Geometry: final body of the model. Coordinates: model frame, mm. A direction names the side the tool comes from. Coordinates: 2 decimals unless noted, no trailing zeros. Write each loop counter-clockwise with the first axis right and the second up, starting at its lowest first coordinate (ties: lowest second). Pieces come first, ordered by that corner, then holes. Notation, with made-up numbers: M 66,43.5 L 90,43.5 A18 ccw 90,57.5 Z; hole C 26.5,29.5 d8. An arc over 180 degrees is marked long. Write item = value, one per line. Start each with the question number.
Item 1: Section B-B on z = 11.5. Give the number of separate pieces and of enclosed holes in the cut face, plus the area to 3 significant figures.
Item 2: Section D-D on x = 18.5. Output: boundary loops of the cut face in (y, z).
Item 3: Pull-direction query (Y, two-part tool) for faces 1 (the flat face through (-7, 13, 15.773)), 2 (the cylindrical face through (29.887, 13.298, 7.776)), 3 (the cylindrical face through (-1.58, 19.27, 7.78)); classes: +Y half, -Y half, draft (parallel to the pull), parting line (faces both ways), or undercut.
Item 4: Reachability of faces 4 (the flat face through (-32, 17.234, 20)), 5 (the flat face through (-14.267, 36.465, 7.776)) from +Z, -Z, +X, -X, +Y, -Y: full face, straight path, thin tool, end or side. Return the list, or none.
Item 5: First-contact query: pin 1 Ø1.5 at (y, z) = (35, 12.5) entering from -X; pin 2 Ø2 at (x, y) = (15.5, 28) entering from +Z; pin 3 Ø5.5 at (x, z) = (-33, 19.5) entering from -Y; pin 4 Ø12 at (x, y) = (-44.5, 19) entering from -Z. Flat tips, straight axial feed; report the tip coordinate or a pass-through.
Item 6: Ray query, L1, parallel to X at y = 13, z = 27; L2, parallel to X at y = 14, z = 7.5; L3, parallel to Z at x = -22, y = -3. Return the intervals inside material, ascending. Write a range as [from, to].
from build123d import *

# Parameters (mm, degrees)
F1_DEPTH = 40.2336
F0_R     = 10.16
F2_DEPTH = 15.7734
F3_R     = 3.302


with BuildPart() as f1:
    # F0 (on Top) → F1 (new body)
    with BuildSketch(Plane.XY):
        with BuildLine():
            ThreePointArc((-42.827169, -15.683244), (-26.084127, -5.852856), (-19.488047, 12.407968))
            ThreePointArc((-19.488047, 12.407968), (-26.084127, 30.668792), (-42.827169, 40.49918))
            ThreePointArc((-42.827169, 40.49918), (-76.638047, 12.407968), (-42.827169, -15.683244))
        make_face()
        with BuildLine():
            ThreePointArc((-34.615282, 7.581968), (-62.350547, 12.407968), (-34.615282, 17.233968))
            Line((-34.615282, 17.233968), (-29.533747, 17.233968))
            Line((-29.533747, 17.233968), (-29.533747, 7.581968))
            Line((-29.533747, 7.581968), (-34.615282, 7.581968))
        make_face(mode=Mode.SUBTRACT)
    extrude(amount=F1_DEPTH)

    # F0 (on Top) → F2 (join)
    with BuildSketch(Plane.XY):
        with BuildLine():
            ThreePointArc((-42.827169, -15.683244), (-26.084127, -5.852856), (-19.488047, 12.407968))
            ThreePointArc((-19.488047, 12.407968), (-26.084127, 30.668792), (-42.827169, 40.49918))
            ThreePointArc((-42.827169, 40.49918), (-76.638047, 12.407968), (-42.827169, -15.683244))
        make_face()
        with BuildLine():
            ThreePointArc((-34.615282, 7.581968), (-62.350547, 12.407968), (-34.615282, 17.233968))
            Line((-34.615282, 17.233968), (-29.533747, 17.233968))
            Line((-29.533747, 17.233968), (-29.533747, 7.581968))
            Line((-29.533747, 7.581968), (-34.615282, 7.581968))
        make_face(mode=Mode.SUBTRACT)
        with BuildLine():
            ThreePointArc((-42.827169, 40.49918), (-26.084127, 30.668792), (-19.488047, 12.407968))
            ThreePointArc((-19.488047, 12.407968), (-26.084127, -5.852856), (-42.827169, -15.683244))
            Line((-42.827169, -15.683244), (13.505259, -5.183529))
            ThreePointArc((13.505259, -5.183529), (29.890809, 13.679218), (13.505259, 32.541964))
            Line((13.505259, 32.541964), (-42.827169, 40.49918))
        make_face()
        with Locations((5.911953, 12.407968)):
            Circle(F0_R, mode=Mode.SUBTRACT)
    extrude(amount=F2_DEPTH)

    # F3
    f3_edges = [f1.edges().sort_by_distance(p)[0] for p in [
        (-53.298926, 40.49918, 40.2336),
    ]]
    fillet(f3_edges, radius=F3_R)


solid = f1.part
Responses:
q1.separate_pieces = 1
q1.enclosed_holes = 2
q1.area = 3,680 mm²
q2.outline = M -3.76,0 L 31.12,0 L 31.12,15.77 L -3.76,15.77 Z
q3.face_1 = draft
q3.face_2 = parting line
q3.face_3 = undercut
q4.face_4 = +Z, -Z
q4.face_5 = +Z, -Z, +X, +Y
q5.pin_1 = -66.49
q5.pin_2 = 15.77
q5.pin_3 = -13.38
q5.pin_4 = through
q6.L1 = [-76.63, -62.34], [-29.53, -19.49]
q6.L2 = [-76.59, -62.26], [-29.53, -4.12], [15.95, 29.89]
q6.L3 = [0, 15.77]
